Design review of the part built by this model. Coordinates are the model's own, in mm. A direction names the side the tool comes from. Coordinates: 2 decimals unless noted, no trailing zeros. Loops run counter-clockwise (first coordinate to the right, second up) from the corner with the lowest first, then second, coordinate; pieces in that order, holes last. Notation, with made-up numbers: M -38,85 L 1,85 A13 cw 1,94 Z; hole C -30.5,70 d4. An arc over 180 degrees is marked long. Put each result on its own line as item: value. Start each with the question number.
(1) Clearance check with flat-ended pins moving along their axes: pin 1 (2 mm diameter, centred on y = 2, z = -4.5, fed in from +X); pin 2 (1 mm diameter, centred on x = -42.5, y = 3, fed in from -Z). State where each tip first meets the part, or that it passes through.
(2) For faces 1 (the cylindrical face through (2.68, 1.97, -43.82)), 2 (the flat face through (1, 4, 12)), list the 3-axis set-ups (+Z, -Z, +X, -X, +Y, -Y) from which the entire face can be reached by the end or side of a thin tool; tool diameter is ignored.
(3) The part is to be moulded in two halves that separate along X. For faces 3 (the cylindrical face through (2.64, 1.97, -59.94)), 4 (the cylindrical face through (-5.25, 1.97, 20.83)), 5 (the flat face through (1, 0, 12)), say which applies: +X half, -X half, draft (parallel to the pull), parting line (faces both ways), or undercut.
(4) Take a section at B-B, the plane z = -28.5. Give the boundary of the cut face in (x, y), then the cut area to 3 significant figures.
(5) Take a section at D-D, the plane y = 1.95. Count the separate pieces of the cut face and the enclosed holes in it, then the cut area to 3 significant figures.
(6) Take a section at A-A, the plane x = 8. Give the boundary of the cut face in (y, z).
(7) Take a section at C-C, the plane z = 11. Give the boundary of the cut face in (x, y) (3 decimals), then the cut area to 3 significant figures.
(8) For probe 1 along Z at (x, y) = (1, 0.8); probe 2 along X at (y, z) = (2.95, -1); probe 3 along X at (y, z) = (2.3, -21), list the stretches that pass through material, from the lowest coordinate up. Write a range as [from, to].
```python
from build123d import *

# Parameters (mm, degrees)
SKETCH_3_R           = 60
SKETCH_3_R_2         = 1.052935028
SKETCH_3_R_3         = 1.5
SKETCH_3_R_4         = 1.55
EXTRUDE_4_DEPTH      = 4
CUT_EXTRUDE_15_DEPTH = 4
SKETCH_3_22_R        = 1.55
CUT_EXTRUDE_23_DEPTH = 10
SKETCH_3_23_R        = 1.052935028
CUT_EXTRUDE_24_DEPTH = 10


with BuildPart() as part:
    # 草图3 → 凸台-拉伸4 (new body)
    with BuildSketch(Plane(origin=(0, 0, 0), x_dir=(1, 0, 0), z_dir=(0, 1, 0))):
        with Locations(Location((0, 0, 0), (0, 0, 270))):
            Circle(SKETCH_3_R)
        with Locations(Location((-46.641583195, -34.475537952, 0), (0, 0, 270))):
            Circle(SKETCH_3_R_2, mode=Mode.SUBTRACT)
        with Locations(Location((-13.569076992, -56.390426045, 0), (0, 0, 270))):
            Circle(SKETCH_3_R_2, mode=Mode.SUBTRACT)
        with BuildLine():
            ThreePointArc((-44.889569885, -22.021047103), (-39.209954392, -19.560908928), (-33.307112163, -17.698983687))
            Line((-33.307112163, -17.698983687), (21.609631998, -30.913452559))
            ThreePointArc((21.609631998, -30.913452559), (26.019303967, -35.256850436), (29.958048994, -40.031428909))
            ThreePointArc((29.958048994, -40.031428909), (-11.697480165, -48.612436246), (-44.889569885, -22.021047103))
        make_face(mode=Mode.SUBTRACT)
        with Locations(Location((-4.678992066, -19.444974498, 0), (0, 0, 270))):
            Circle(SKETCH_3_R_3, mode=Mode.SUBTRACT)
        with Locations(Location((-3.50924405, -14.583730874, 0), (0, 0, 270))):
            Circle(SKETCH_3_R_4, mode=Mode.SUBTRACT)
        with Locations(Location((-4.794834481, -1.417590314, 0), (0, 0, 270))):
            Circle(SKETCH_3_R_4, mode=Mode.SUBTRACT)
        with Locations(Location((25.852551139, -51.919607083, 0), (0, 0, 270))):
            Circle(SKETCH_3_R_2, mode=Mode.SUBTRACT)
        with Locations(Location((53.177483273, -23.155026944, 0), (0, 0, 270))):
            Circle(SKETCH_3_R_2, mode=Mode.SUBTRACT)
        with Locations(Location((-10.875259394, 10.330959932, 0), (0, 0, 270))):
            Circle(SKETCH_3_R_4, mode=Mode.SUBTRACT)
        with Locations(Location((-14.500345858, 13.774613243, 0), (0, 0, 270))):
            Circle(SKETCH_3_R_3, mode=Mode.SUBTRACT)
        with BuildLine():
            ThreePointArc((15.967019236, 34.171216556), (17.523676152, 40.161803442), (19.689209887, 45.960145931))
            ThreePointArc((19.689209887, 45.960145931), (47.948344812, 14.175903139), (41.515571152, -27.864984334))
            ThreePointArc((41.515571152, -27.864984334), (36.545221249, -24.176362121), (31.981325576, -19.995313417))
            Line((31.981325576, -19.995313417), (15.967019236, 34.171216556))
        make_face(mode=Mode.SUBTRACT)
        with Locations(Location((55.620079982, 16.444047642, 0), (0, 0, 270))):
            Circle(SKETCH_3_R_2, mode=Mode.SUBTRACT)
        with Locations(Location((32.037423118, 48.34876958, 0), (0, 0, 270))):
            Circle(SKETCH_3_R_2, mode=Mode.SUBTRACT)
        with Locations(Location((-42.05100299, 39.946378404, 0), (0, 0, 270))):
            Circle(SKETCH_3_R_2, mode=Mode.SUBTRACT)
        with Locations(Location((-6.535900078, 57.630564895, 0), (0, 0, 270))):
            Circle(SKETCH_3_R_2, mode=Mode.SUBTRACT)
        with Locations(Location((14.384503444, 4.252770942, 0), (0, 0, 270))):
            Circle(SKETCH_3_R_4, mode=Mode.SUBTRACT)
        with Locations(Location((19.179337925, 5.670361256, 0), (0, 0, 270))):
            Circle(SKETCH_3_R_3, mode=Mode.SUBTRACT)
    extrude(amount=EXTRUDE_4_DEPTH)

    # 草图3<17> → 切除-拉伸15 (cut)
    with BuildSketch(Plane(origin=(0, 0, 0), x_dir=(1, 0, 0), z_dir=(0, 1, 0))):
        with BuildLine():
            Line((1.325786588, 37.694297104), (-37.576651234, -3.257763997))
            ThreePointArc((-37.576651234, -3.257763997), (-43.542980118, -4.904953006), (-49.647258882, -5.928717023))
            ThreePointArc((-49.647258882, -5.928717023), (-36.250864646, 34.436533107), (3.373998733, 49.886031437))
            ThreePointArc((3.373998733, 49.886031437), (2.664733143, 43.737271049), (1.325786588, 37.694297104))
        make_face()
    extrude(amount=CUT_EXTRUDE_15_DEPTH, mode=Mode.SUBTRACT)

    # 草图3<22> → 切除-拉伸23 (cut)
    with BuildSketch(Plane(origin=(0, 0, 0), x_dir=(1, 0, 0), z_dir=(0, 1, 0))):
        with Locations(Location((0, 0, 0), (0, 0, 270))):
            Circle(SKETCH_3_22_R)
    extrude(amount=CUT_EXTRUDE_23_DEPTH, mode=Mode.SUBTRACT)

    # 草图3<23> → 切除-拉伸24 (cut)
    with BuildSketch(Plane(origin=(0, 0, 0), x_dir=(1, 0, 0), z_dir=(0, 1, 0))):
        with Locations(Location((-57.889974257, 3.570837502, 0), (0, 0, 270))):
            Circle(SKETCH_3_23_R)
    extrude(amount=CUT_EXTRUDE_24_DEPTH, mode=Mode.SUBTRACT)


solid = part.part
```
Computed values:
1. pin 1: stops at x = 59.9
1. pin 2: stops at z = -42.85
2. face 1: +Y, -Y
2. face 2: +Z, -Z, +X, -X, +Y
3. face 3: parting line
3. face 4: undercut
3. face 5: draft
4. outline: M -52.8,0 L -41.08,0 L -41.08,4 L -52.8,4 Z; M -7.41,0 L 17.64,0 L 17.64,4 L -7.41,4 Z; M 41.08,0 L 52.8,0 L 52.8,4 L 41.08,4 Z
4. area: 194 mm^2
5. separate pieces: 1
5. enclosed holes: 20
5. area: 6,920 mm^2
6. outline: M 0,-59.46 L 4,-59.46 L 4,27.64 L 0,27.64 Z; M 0,49.36 L 4,49.36 L 4,59.46 L 0,59.46 Z
7. outline: M -58.983,0 L 29.322,0 L 29.322,4 L -58.983,4 Z; M 48.775,0 L 58.983,0 L 58.983,4 L 48.775,4 Z
7. area: 394 mm^2
8. probe 1: z = [-59.99, -49.99], [-37.35, -1.18], [1.18, 25.95], [49.99, 59.99]
8. probe 2: x = [-59.99, -49.99], [-33.53, -1.18], [1.18, 25.77], [49.99, 59.99]
8. probe 3: x = [-56.2, -45.38], [-14.53, 19.86], [45.38, 56.2]
